```python
from build123d import *

# Parameters (mm, degrees)
SKETCH_1_R          = 6
EXTRUDE_1_DEPTH     = 5
FILLET_1_R          = 5
FILLET_2_R          = 75
FILLET_3_R          = 5
SKETCH_3_R          = 2.6
CUT_EXTRUDE_1_DEPTH = 160.415234704


with BuildPart() as part:
    # Эскиз1 → Бобышка-Вытянуть1 (new body)
    with BuildSketch(Plane(origin=(0, 0, 0), x_dir=(0, 0, -1), z_dir=(1, 0, 0))):
        with BuildLine():
            Line((126.237664014, 58.886284382), (98.821729218, -16.438377404))
            Line((98.821729218, -16.438377404), (-151.178270782, -25.884067346))
            Line((-151.178270782, -25.884067346), (-77.345590471, -3.080194644))
            Line((-77.345590471, -3.080194644), (-77.345590471, -13.087329783))
            Line((-77.345590471, -13.087329783), (75.539410437, -7.310912522))
            Line((75.539410437, -7.310912522), (90.975731778, 35.100031802))
            ThreePointArc((90.975731778, 35.100031802), (108.905022115, 46.550907327), (126.237664014, 58.886284382))
        make_face()
        with Locations((103.870185422, 30.698515365)):
            Circle(SKETCH_1_R, mode=Mode.SUBTRACT)
    extrude(amount=EXTRUDE_1_DEPTH)

    # Скругление1
    fillet_1_edges = [part.edges().sort_by_distance(p)[0] for p in [
        (2.5, -13.087329783, 77.345590471),
    ]]
    fillet(fillet_1_edges, radius=FILLET_1_R)

    # Скругление2
    # the kernel refuses this fillet: 75 mm, written as the material it adds along each edge
    with BuildSketch(Plane(origin=(0, -7.310912522, -75.539410437), x_dir=(0, -0.037755820465347284, 0.9992869948223027), z_dir=(1, 0, 0))) as fillet_2_piece_1:
        with BuildLine():
            CenterArc((50.223853574, -75), FILLET_2_R, 90, 63.724056715)
            Line((-17.026575163, -41.797894123), (0, 0))
            Line((0, 0), (50.223853574, 0))
        make_face()
    extrude(amount=5)
    # the kernel refuses this fillet: 75 mm, written as the material it takes off along each edge
    with BuildSketch(Plane(origin=(-126.080854452, -16.438377404, -98.821729218), x_dir=(0, -0.03775582046534733, 0.9992869948223025), z_dir=(1, 0, 0))) as fillet_2_2_piece_1:
        with BuildLine():
            CenterArc((FILLET_2_R * 0.672431223743, -FILLET_2_R), FILLET_2_R, 90, 67.836236553)
            Line((-FILLET_2_R * 0.253678140212, -FILLET_2_R * 0.622744852924), (0, 0))
            Line((0, 0), (FILLET_2_R * 0.672431223743, 0))
        make_face()
    extrude(amount=257.161708904, mode=Mode.SUBTRACT)

    # Скругление3
    fillet_3_edges = [part.edges().sort_by_distance(p)[0] for p in [
        (2.5, 58.886284382, -126.237664014),
    ]]
    fillet(fillet_3_edges, radius=FILLET_3_R)

    # Эскиз3 → Вырез-Вытянуть1 (cut, through all)
    with BuildSketch(Plane(origin=(5, 0, 0), x_dir=(0, 0, -1), z_dir=(1, 0, 0))):
        with Locations((-23.402722319, -16.052786924)):
            Circle(SKETCH_3_R)
    extrude(amount=-CUT_EXTRUDE_1_DEPTH, mode=Mode.SUBTRACT)


solid = part.part
```
Model file for the job. Use its own axes, mm. A direction names the side the tool comes from. Give positions to 0.01 mm unless a question says otherwise; leave off trailing zeros. Write each loop counter-clockwise with the first axis right and the second up, starting at its lowest first coordinate (ties: lowest second). Pieces come first, ordered by that corner, then holes. Notation, with made-up numbers: (22.5, 14) -> (33.5, 14) arc R20 cw to (33.5, 50) -> close; hole circle Ø11 at (66.25, 50). An arc over 180 degrees is marked (long way). Use CSV: the item, a comma, the result in double quotes. Start each with the question number.
1) Drill centre lines: L1, parallel to Y at x = 3, z = -106.5; L2, parallel to Z at x = 3.85, y = 33.5; L3, parallel to Z at x = 2.05, y = 29. Where is each one in solid material? Low to high.
2) Cut at B-B on y = 15. List the corners of the cut face in (x, z), plus the area to 3 significant figures.
3) Cut at A-A on x = 1.55. List the corners of the cut face in (y, z).
4) Pin check, flat tips, straight feed: P1, Ø1.5, axis at x = 2, y = 4, coming from the -Z side; P2, Ø2, axis at x = 1, y = 34, coming from the -Z side; P3, Ø11, axis at y = 30.7, z = -103.87, coming from the -X side; P4, Ø1.4, axis at x = 3.5, y = -6.5, coming from the -Z side. Stop position of each tip, or through.
5) Cut at C-C on z = -1. List the corners of the cut face in (x, y), plus the area to 3 significant figures.
6) Tool access for faces 5 (the flat face through (2.465, -11.075, 24.085)), 6 (the flat face through (2.465, -14.642, 114.779)): list every direction of +Z, -Z, +X, -X, +Y, -Y with a clear straight run to the whole face (end or side of a thin tool).
7) Two-plate mould, pull along Y, no slides. Class faces 1 (the cylindrical face through (2.465, 32.501, -109.593)), 2 (the cylindrical face through (2.465, 3.256, -64.002)), 3 (the cylindrical face through (2.54, -17.63, 25.47)), 4 (the cylindrical face through (2.535, 49.344, -118.967)): released by +Y, released by -Y, zero draft, split by the parting line, or undercut.
Final values:
1,L1,"y = 12.84 to 25.31, 36.09 to 44.94"
1,L2,"z = -117 to -109.18, -98.56 to -90.24"
1,L3,"z = -115.33 to -109.62, -98.12 to -87.9"
2,outline,"(0, -108) -> (5, -108) -> (5, -77.75) -> (0, -77.75) -> close"
2,area,"151 mm2"
3,outline,"(-25.88, 151.18) -> (-18.34, -48.43) arc R75 ccw to (30.95, -116.07) -> (43.62, -120.68) arc R5 ccw to (49.44, -113.14) arc R424.19 cw to (35.1, -90.98) arc R75 cw to (-9.21, -25.35) -> (-12.89, 72.16) arc R5 cw to (-7.89, 77.35) -> (-3.08, 77.35) -> close; hole circle Ø5.2 at (-16.05, 23.4); hole circle Ø12 at (30.7, -103.87)"
4,P1,"stops at z = -99.78"
4,P2,"stops at z = -117.54"
4,P3,"passes through"
4,P4,"stops at z = -87.2"
5,outline,"(0, -20.13) -> (5, -20.13) -> (5, -10.13) -> (0, -10.13) -> close"
5,area,"50.0 mm2"
6,face 5,"+X, -X, +Y"
6,face 6,"+Z, +X, -X, +Y"
7,face 1,"undercut"
7,face 2,"released by +Y"
7,face 3,"undercut"
7,face 4,"split by the parting line"
